```python
from build123d import *

# Parameters (mm, degrees)
EXTRUDE_1_DEPTH     = 3
SKETCH_2_W          = 30
SKETCH_2_H          = 3
EXTRUDE_2_DEPTH     = 10
SKETCH_4_W          = 5
SKETCH_4_H          = 14
CUT_EXTRUDE_1_DEPTH = 10


with BuildPart() as part:
    # Эскиз1 → Бобышка-Вытянуть1 (new body)
    with BuildSketch(Plane(origin=(0, 0, 0), x_dir=(1, 0, 0), z_dir=(0, 1, 0))):
        Polygon((-15, -50), (15, -50), (15, -30.397249725), (12, -30.397249725), (12, -15.597249725), (15, -15.597249725), (15, 15.597249725), (12, 15.597249725), (12, 30.397249725), (15, 30.397249725), (15, 50), (-15, 50), (-15, 30.397249725), (-12, 30.397249725), (-12, 15.597249725), (-15, 15.597249725), (-15, -15.597249725), (-12, -15.597249725), (-12, -30.397249725), (-15, -30.397249725), align=None)
    extrude(amount=EXTRUDE_1_DEPTH)

    # Эскиз2 → Бобышка-Вытянуть2 (add)
    with BuildSketch(Plane(origin=(0, 0, -50), x_dir=(-1, 0, 0), z_dir=(0, 0, -1))):
        with Locations((0, 1.5)):
            Rectangle(SKETCH_2_W, SKETCH_2_H)
    extrude(amount=EXTRUDE_2_DEPTH)

    # Эскиз4 → Вырез-Вытянуть1 (cut)
    with BuildSketch(Plane(origin=(0, 3, 0), x_dir=(1, 0, 0), z_dir=(0, 1, 0))):
        with Locations((0, -40.597249725)):
            Rectangle(SKETCH_4_W, SKETCH_4_H)
    extrude(amount=-CUT_EXTRUDE_1_DEPTH, mode=Mode.SUBTRACT)


solid = part.part
```
Can you work these out from the model? Positions are in its coordinate system, mm. A direction names the side the tool comes from. Give positions to 0.01 mm unless a question says otherwise; leave off trailing zeros. Order: outer loops, then holes, each group sorted by start corner. A loop starts at its lowest first (then second) coordinate and runs counter-clockwise, first axis right, second up. Notation, with made-up numbers: M 65.25,43.25 L 98.25,43.25 A13 cw 98.25,51.25 Z; hole C 16,59 d1. An arc over 180 degrees is marked long. One line per item, written item: value.
1) For P1, Ø1.5, axis at x = 11, z = 36, coming from the -Y side; P2, Ø0.9, axis at y = 2, z = -24, coming from the -X side, each with a flat end and sliding along its axis, tell me the tip position at first contact or that it passes through.
Answer sheet:
P1: stops at y = 0
P2: stops at x = -12
2) We'd pull the mould along Z, two halves only. Please class faces 1 (the face through (12, 1, 23)), 2 (the face through (0, 1, 50)), 3 (the face through (15, 1, 40)): released by +Z, released by -Z, zero draft, split by the parting line, or undercut.
Answer sheet:
face 1: undercut
face 2: released by +Z
face 3: zero draft
3) Please list where these lines run through material, in increasing order: line 1 along Z through (x, y) = (0, 1.7); line 2 along X through (y, z) = (2.7, 39); line 3 along X through (y, z) = (1.9, 28.5).
Answer sheet:
line 1: z = -60 to 33.6, 47.6 to 50
line 2: x = -15 to -2.5, 2.5 to 15
line 3: x = -12 to 12
4) I want a section at B-B, the plane z = 21.5. List the corners of the cut face in (x, y) for me, plus the area to 3 significant figures.
Answer sheet:
outline: M -12,0 L 12,0 L 12,3 L -12,3 Z
area: 72.0 mm^2
5) I want a section at A-A, the plane y = 1.45. List the corners of the cut face in (x, z) for me.
Answer sheet:
outline: M -15,-60 L 15,-60 L 15,-30.4 L 12,-30.4 L 12,-15.6 L 15,-15.6 L 15,15.6 L 12,15.6 L 12,30.4 L 15,30.4 L 15,50 L -15,50 L -15,30.4 L -12,30.4 L -12,15.6 L -15,15.6 L -15,-15.6 L -12,-15.6 L -12,-30.4 L -15,-30.4 Z; hole M -2.5,33.6 L 2.5,33.6 L 2.5,47.6 L -2.5,47.6 Z
6) On a 3-axis mill with a long thin cutter (end or side, diameter ignored), from which of +Z, -Z, +X, -X, +Y, -Y can I reach the whole of each face in a straight line? I mean faces 4 (the face through (-13, 1, 30.397)), 5 (the face through (14, 1, -15.597)), 6 (the face through (-15, 1, -45)), 7 (the face through (15, 1, -45)), 8 (the face through (0, 2, 47.597)). Say none if no direction works.
Answer sheet:
face 4: -X, +Y, -Y
face 5: +X, +Y, -Y
face 6: +Z, -Z, -X, +Y, -Y
face 7: +Z, -Z, +X, +Y, -Y
face 8: +Y, -Y
